```python
from build123d import *

# Parameters (mm, degrees)
SKETCH_3_R                = 2.825
CUT_EXTRUDE_2_DEPTH       = 35
SKETCH_16_W               = 5.008881277
SKETCH_16_H               = 1
EXTRUDE_2_DEPTH           = 30
SKETCH_19_W               = 0.959066555
SKETCH_19_H               = 0.511502163
EXTRUDE_3_DEPTH           = 30
SKETCH_24_W               = 45.827715764
SKETCH_24_H               = 4
CUT_EXTRUDE_8_DEPTH       = 9
SKETCH_25_R               = 1.43
CUT_EXTRUDE_9_DEPTH       = 22
SKETCH_27_R               = 2
SKETCH_27_R_2             = 1
EXTRUDE_2_2_DEPTH         = 4
SKETCH_28_R               = 1.43
CUT_EXTRUDE_11_DEPTH      = 25
CUT_EXTRUDE_12_DEPTH      = 12.15
CUT_EXTRUDE_12_DEPTH_BACK = 35
SKETCH_29_W               = 9
SKETCH_29_H               = 3.960677992
SKETCH_30_R               = 47
SKETCH_30_R_2             = 26
CUT_EXTRUDE_1_DEPTH       = 10


with BuildPart() as part:
    # 草圖1 → 旋轉1 (revolve)
    with BuildSketch(Plane.XY, mode=Mode.PRIVATE) as revolve_1_sk:
        Polygon((0, 0), (0, 44), (9.74, 44), (21.74, 34.418858447), (28.74, 34.418858447), (40.74, 44), (50.48, 44), (50.48, 34.418858447), (60.48, 34.418858447), (60.48, 0), align=None)
    revolve(revolve_1_sk.sketch.rotate(Axis((-743.15639781, 0, 0), (1, 0, 0)), 90), axis=Axis((-743.15639781, 0, 0), (1, 0, 0)))

    # 草圖3 → 除料-伸長2 (cut)
    with BuildSketch(Plane(origin=(60.48, 0, 0), x_dir=(0, 0, -1), z_dir=(1, 0, 0))):
        Circle(SKETCH_3_R)
    extrude(amount=-CUT_EXTRUDE_2_DEPTH, mode=Mode.SUBTRACT)

    # 草圖16 → Extrude 2 (add)
    with BuildSketch(Plane(origin=(60.48, 0, 0), x_dir=(0, 0, -1), z_dir=(1, 0, 0))):
        with Locations((-0.105543204, 2.350977924)):
            Rectangle(SKETCH_16_W, SKETCH_16_H)
    extrude(amount=-EXTRUDE_2_DEPTH)

    # 草圖19 → 填料-伸長3 (add)
    with BuildSketch(Plane(origin=(60.48, 0, 0), x_dir=(0, 0, -1), z_dir=(1, 0, 0))):
        with Locations((-0.084116996, 2.673942601)):
            Rectangle(SKETCH_19_W, SKETCH_19_H)
    extrude(amount=-EXTRUDE_3_DEPTH)

    # 草圖24 → 除料-伸長8 (cut)
    with BuildSketch(Plane(origin=(60.48, 0, 0), x_dir=(0, 0, -1), z_dir=(1, 0, 0))):
        with Locations((10.762797737, 9.109197083)):
            Rectangle(SKETCH_24_W, SKETCH_24_H)
    extrude(amount=-CUT_EXTRUDE_8_DEPTH, mode=Mode.SUBTRACT)

    # 草圖25 → 除料-伸長9 (cut)
    with BuildSketch(Plane(origin=(0, 22, 0), x_dir=(1, 0, 0), z_dir=(0, 1, 0))):
        with Locations(Location((29.956679037, 0, 0), (0, 0, 270))):
            Circle(SKETCH_25_R)
    extrude(amount=-CUT_EXTRUDE_9_DEPTH, mode=Mode.SUBTRACT)

    # 草圖27 → Extrude 2 2 (add)
    with BuildSketch(Plane.XY):
        with Locations((25.24, 35.418858447)):
            Circle(SKETCH_27_R)
        with Locations((25.24, 35.418858447)):
            Circle(SKETCH_27_R_2, mode=Mode.SUBTRACT)
    extrude(amount=EXTRUDE_2_2_DEPTH)

    # 草圖28 → 除料-伸長11 (cut)
    with BuildSketch(Plane(origin=(0, 35, 0), x_dir=(1, 0, 0), z_dir=(0, 1, 0))):
        with Locations(Location((55.48, 0, 0), (0, 0, 270))):
            Circle(SKETCH_28_R)
    extrude(amount=-CUT_EXTRUDE_11_DEPTH, mode=Mode.SUBTRACT)

    # 草圖29 → 除料-伸長12 (cut, two sides: drawn at the far end of the back side and taken through both)
    with BuildSketch(Plane.XY.offset(-CUT_EXTRUDE_12_DEPTH_BACK)):
        with Locations((55.98, 5.128858087)):
            Rectangle(SKETCH_29_W, SKETCH_29_H)
    extrude(amount=CUT_EXTRUDE_12_DEPTH + CUT_EXTRUDE_12_DEPTH_BACK, mode=Mode.SUBTRACT)

    # 草圖30 → 除料-伸長-薄件1 (cut)
    with BuildSketch(Plane(origin=(60.48, 0, 0), x_dir=(0, 0, -1), z_dir=(1, 0, 0))):
        Circle(SKETCH_30_R)
        Circle(SKETCH_30_R_2, mode=Mode.SUBTRACT)
    extrude(amount=-CUT_EXTRUDE_1_DEPTH, mode=Mode.SUBTRACT)


solid = part.part
```
Design review of the part built by this model. Coordinates are the model's own, in mm. A direction names the side the tool comes from. Give positions to 0.01 mm unless a question says otherwise; leave off trailing zeros. Loops run counter-clockwise (first coordinate to the right, second up) from the corner with the lowest first, then second, coordinate; pieces in that order, holes last. Notation, with made-up numbers: M 62.25,-5.75 L 106.25,-5.75 A21 ccw 106.25,30.25 Z; hole C 11,81 d7. An arc over 180 degrees is marked long. Return JSON: item names as keys, results as strings. Group by question number.
Item 1: We need section A-A (x = 55.48). Give the number of separate pieces and of enclosed holes in the cut face, and give its area (3 significant figures).
Item 2: We need section C-C (x = 33). Give the boundary of the cut face in (y, z) (3 decimals), and give its area (3 significant figures).
Item 3: We need section D-D (x = 12). Give the boundary of the cut face in (y, z).
Item 4: Mouldability with a two-part tool opening along Y and no side actions: class faces 6 (the flat face through (25, 37, 4)), 7 (the flat face through (46, 1.851, 0)), 8 (the conical face through (21.157, 34.055, -7.562)) as released by +Y, released by -Y, zero draft, split by the parting line, or undercut.
Item 5: Insertion check: pin 1 Ø8 at (x, z) = (37.5, 25) entering from -Y; pin 2 Ø6 at (x, z) = (48.5, 28) entering from +Y; pin 3 Ø2.5 at (x, y) = (25, 36) entering from +Z. Each pin has a flat end and moves straight along its axis. Give the tip position at first contact, or say it passes through.
Item 6: Tool access review of faces 1 (the cylindrical face through (56.898, 18.659, -0.186)), 2 (the flat face through (25.48, 0, 0)), 3 (the flat face through (56, 9, 12.151)), 4 (the flat face through (60.48, -5, 0)), 5 (the flat face through (50.48, 19, 19)): name each direction out of +Z, -Z, +X, -X, +Y, -Y from which nothing blocks a thin tool from reaching the whole face with its end or side.
Item 7: For probe 1 along X at (y, z) = (15.75, 0); probe 2 along Y at (x, z) = (48, 0) (3 decimals); probe 3 along X at (y, z) = (8.75, 0), list the stretches that pass through material, from the lowest coordinate up.
Item 8: We need section B-B (y = 0). Give the boundary of the cut face in (x, z) (3 decimals).
Output:
{
 "1": {"separate pieces": "2", "enclosed holes": "1", "area": "1,760 mm^2"},
 "2": {"outline": "C 0,0 d75.64; hole M 1.851,-2.134 L 1.851,2.134 A2.825 ccw long Z", "area": "4,470 mm^2"},
 "3": {"outline": "C 0,0 d84.39"},
 "4": {"face 6": "zero draft", "face 7": "undercut", "face 8": "split by the parting line"},
 "5": {"pin 1": "stops at y = -37.72", "pin 2": "stops at y = 36.21", "pin 3": "stops at z = 4"},
 "6": {"face 1": "+Y", "face 2": "none", "face 3": "-Z, +X", "face 4": "+Z, -Z, +X, +Y, -Y", "face 5": "+X"},
 "7": {"probe 1": "x = 0 to 28.53, 31.39 to 54.05, 56.91 to 60.48", "probe 2": "y = -44 to -2.825, 1.851 to 44", "probe 3": "x = 0 to 28.53, 31.39 to 51.48"},
 "8": {"outline": "M 0,-44 L 9.74,-44 L 21.74,-34.419 L 28.74,-34.419 L 40.74,-44 L 50.48,-44 L 50.48,-26 L 60.48,-26 L 60.48,-2.825 L 25.48,-2.825 L 25.48,2.825 L 60.48,2.825 L 60.48,26 L 50.48,26 L 50.48,44 L 40.74,44 L 28.74,34.419 L 21.74,34.419 L 9.74,44 L 0,44 Z"}
}
